from build123d import *

# Parameters (mm, degrees)
SKETCH1_W                            = 390
SKETCH1_H                            = 90
BOSS_EXTRUDE1_DEPTH                  = 3.175
M4_CLEARANCE_HOLE1_D                 = 4.5
SKETCH4_W                            = 30
SKETCH4_H                            = 70
CUT_EXTRUDE1_DEPTH                   = 201.150145204
FILLET1_R                            = 5
M4_CLEARANCE_HOLE2_D                 = 4.5
MIRROR1_AT_THE_SECOND_PLANE_COPY_1_D = 4.5


with BuildPart() as part:
    # Sketch1 → Boss-Extrude1 (new body)
    with BuildSketch(Plane(origin=(0, 0, 0), x_dir=(0, 0, -1), z_dir=(1, 0, 0))):
        Rectangle(SKETCH1_W, SKETCH1_H)
    extrude(amount=BOSS_EXTRUDE1_DEPTH)

    # M4 Clearance Hole1 (through all)
    with Locations(Plane(origin=(3.175, 0, 0), x_dir=(0, 0, -1), z_dir=(1, 0, 0))):
        with Locations((136.351636823, -15), (-101.563539669, -30), (-51.563539669, -30), (-51.563539669, -15), (86.351636823, -30), (136.351636823, -30)):
            Hole(M4_CLEARANCE_HOLE1_D / 2)

    # Sketch4 → Cut-Extrude1 (cut, through all)
    with BuildSketch(Plane(origin=(3.175, 0, 0), x_dir=(0, 0, -1), z_dir=(1, 0, 0))):
        with Locations((170, 0)):
            Rectangle(SKETCH4_W, SKETCH4_H)
    extrude(amount=-CUT_EXTRUDE1_DEPTH, mode=Mode.SUBTRACT)

    # Fillet1
    fillet1_edges = [part.edges().sort_by_distance(p)[0] for p in [
        (1.5875, 35, -185),
        (1.5875, -35, -185),
        (1.5875, -35, -155),
        (1.5875, 35, -155),
    ]]
    fillet(fillet1_edges, radius=FILLET1_R)

    # M4 Clearance Hole2 (through all)
    with Locations(Plane(origin=(3.175, 0, 0), x_dir=(0, 0, -1), z_dir=(1, 0, 0))):
        with Locations((-186.825, -40)):
            m4_clearance_hole2 = Hole(M4_CLEARANCE_HOLE2_D / 2)

    # Mirror1: M4 Clearance Hole2 across plane
    add(m4_clearance_hole2.mirror(Plane.XY), mode=Mode.SUBTRACT)

    # Mirror1 at the second plane: M4 Clearance Hole2 across plane
    add(m4_clearance_hole2.mirror(Plane.ZX), mode=Mode.SUBTRACT)

    # Mirror1 at the second plane copy 1 (through all)
    with Locations(Plane(origin=(3.175, 0, 0), x_dir=(0, 0, 1), z_dir=(1, 0, 0))):
        with Locations((-186.825, -40)):
            Hole(MIRROR1_AT_THE_SECOND_PLANE_COPY_1_D / 2)


solid = part.part
Design review of the part built by this model. Coordinates are the model's own, in mm. Give positions to 0.01 mm unless a question says otherwise; leave off trailing zeros. Order: outer loops, then holes, each group sorted by start corner. A loop starts at its lowest first (then second) coordinate and runs counter-clockwise, first axis right, second up. Notation, with made-up numbers: (59.5, 44.25) - (86.5, 44.25) arc R22 cw to (86.5, 79.25) - close; hole circle Ø5 at (73.25, 70). An arc over 180 degrees is marked (long way). Write item = value, one per line. Start each with the question number.
Q1. Clearance check with a flat-ended pin moving along its axis: pin 1 Ø2.5 at (y, z) = (-30, -136.35) entering from -X. State where the tip first meets the part, or that it passes through.
Q2. We need section A-A on y = 15. State the section outline as (x, z) points (3 decimals), plus the area to 3 significant figures.
Q3. To check wall thickness, follow L1, parallel to Z at x = 0.3, y = 39.5; L2, parallel to Z at x = 2.9, y = 11.5; L3, parallel to Z at x = 2.7, y = -39. State the ranges of each line that lie inside material, in increasing order. Write a range as from..to.
Q4. We need section B-B on x = 1.4. State how many separate pieces and enclosed holes the cut face has, plus the area to 3 significant figures.
Working result:
q1.pin_1 = through
q2.outline = (0, -195) - (3.175, -195) - (3.175, -185) - (0, -185) - close; (0, -155) - (3.175, -155) - (3.175, 195) - (0, 195) - close
q2.area = 1,140 mm²
q3.L1 = -195..-189.02, -184.63..184.63, 189.02..195
q3.L2 = -195..-185, -155..195
q3.L3 = -195..-188.84, -184.81..184.81, 188.84..195
q4.separate_pieces = 1
q4.enclosed_holes = 11
q4.area = 32,900 mm²
